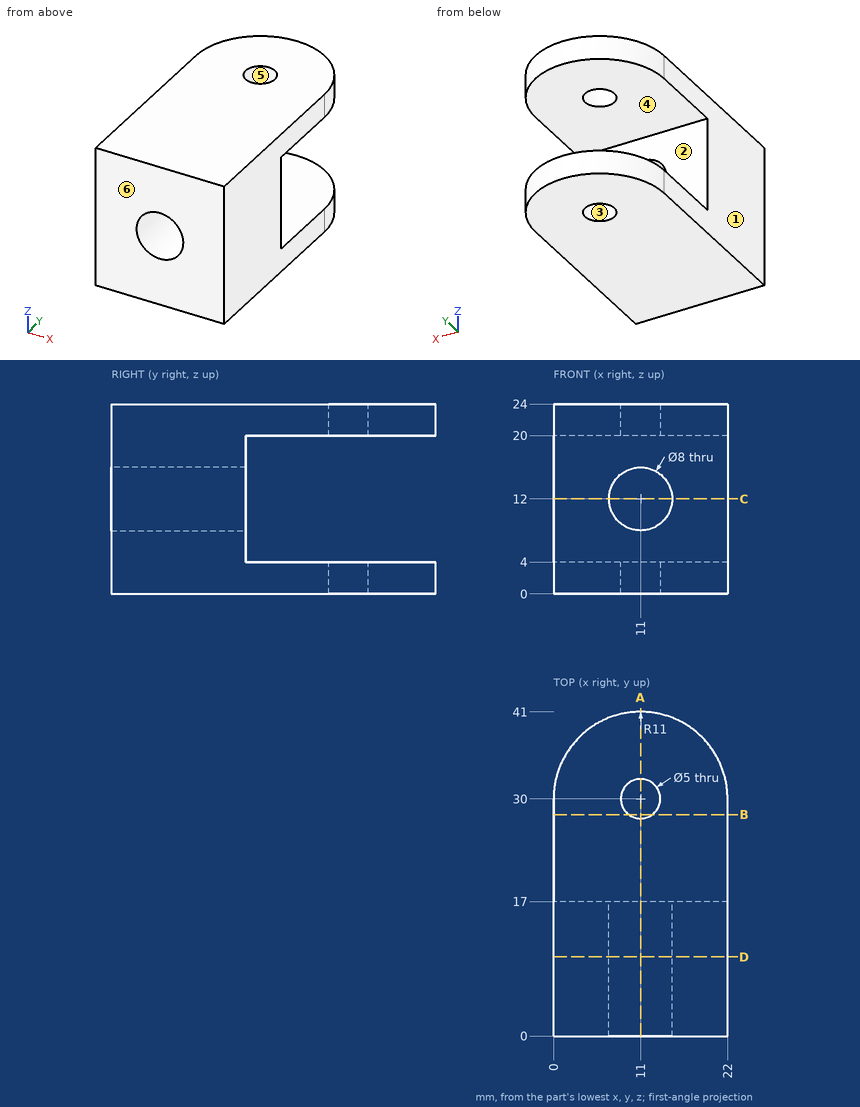
Can you work these out from the drawing? Everything is in mm from the part's minimum corner. A direction names the side the tool comes from. Give positions to 0.01 mm unless a question says otherwise; leave off trailing zeros. Loops run counter-clockwise (first coordinate to the right, second up) from the corner with the lowest first, then second, coordinate; pieces in that order, holes last. Notation, with made-up numbers: (52, 35) -> (75, 35) arc R10 ccw to (75, 46) -> close; hole circle Ø7 at (67, -22). An arc over 180 degrees is marked (long way). Return JSON: item names as keys, results as strings.
Q1. We'd pull the mould along Y, two halves only. Please class the marked faces 3, 4, 5 and 6: released by +Y, released by -Y, zero draft, split by the parting line, or undercut.
Checks:
{"face 3": "undercut", "face 4": "zero draft", "face 5": "undercut", "face 6": "released by -Y"}
Q2. I want a section at B-B, the plane y = 28. List the corners of the cut face in (x, z) for me.
Checks:
{"outline": "(0, 0) -> (9.5, 0) -> (9.5, 4) -> (0, 4) -> close; (0, 20) -> (9.5, 20) -> (9.5, 24) -> (0, 24) -> close; (12.5, 0) -> (22, 0) -> (22, 4) -> (12.5, 4) -> close; (12.5, 20) -> (22, 20) -> (22, 24) -> (12.5, 24) -> close"}
Q3. I need wall thicknesses on probe 1 along X at (y, z) = (11.75, 12); probe 2 along Y at (x, z) = (11, 2.5); probe 3 along Z at (x, y) = (11.25, 20). Which ranges of each line are inside material? Lowest first, please.
Checks:
{"probe 1": "x = 0 to 7, 15 to 22", "probe 2": "y = 0 to 27.5, 32.5 to 41", "probe 3": "z = 0 to 4, 20 to 24"}
Q4. I want a section at C-C, the plane z = 12. List the corners of the cut face in (x, y) for me, then the cut area to 3 significant figures.
Checks:
{"outline": "(0, 0) -> (7, 0) -> (7, 17) -> (0, 17) -> close; (15, 0) -> (22, 0) -> (22, 17) -> (15, 17) -> close", "area": "238 mm2"}
Q5. I want a section at A-A, the plane x = 11. List the corners of the cut face in (y, z) for me, then the cut area to 3 significant figures.
Checks:
{"outline": "(0, 0) -> (27.5, 0) -> (27.5, 4) -> (17, 4) -> (17, 8) -> (0, 8) -> close; (0, 16) -> (17, 16) -> (17, 20) -> (27.5, 20) -> (27.5, 24) -> (0, 24) -> close; (32.5, 0) -> (41, 0) -> (41, 4) -> (32.5, 4) -> close; (32.5, 20) -> (41, 20) -> (41, 24) -> (32.5, 24) -> close", "area": "424 mm2"}
Q6. I want a section at D-D, the plane y = 10. List the corners of the cut face in (x, z) for me, then the cut area to 3 significant figures.
Checks:
{"outline": "(0, 0) -> (22, 0) -> (22, 24) -> (0, 24) -> close; hole circle Ø8 at (11, 12)", "area": "478 mm2"}
Q7. For pin 1 Ø1 at (x, z) = (3.5, 18.5) entering from +Y; pin 2 Ø6.5 at (x, y) = (11, 30) entering from +Z, each with a flat end and sliding along its axis, tell me the tip position at first contact or that it passes through.
Checks:
{"pin 1": "stops at y = 17", "pin 2": "stops at z = 24"}
Q8. On a 3-axis mill with a long thin cutter (end or side, diameter ignored), from which of +Z, -Z, +X, -X, +Y, -Y can I reach the whole of each face in a straight line? I mean the marked faces 1 and 2. Say none if no direction works.
Checks:
{"face 1": "+Z, -Z, -X, +Y, -Y", "face 2": "+X, -X, +Y"}
